from build123d import *

# Parameters (mm, degrees)
SKETCH1_W           = 243.588796282
SKETCH1_H           = 434.599999988
BOSS_EXTRUDE1_DEPTH = 12.7
CUT_EXTRUDE1_REACH  = 273.182
SKETCH2_W           = 141.287862113
SKETCH2_H           = 32.775
CUT_EXTRUDE2_REACH  = 273.182
HOLE1_D             = 3.175
HOLE1_DEPTH         = 38.1
HOLE1_CSINK_D       = 10.16
HOLE1_CSINK_ANGLE   = 82
HOLE1_TIP           = 0.953866233
CUT_EXTRUDE3_REACH  = 273.182
SKETCH6_W           = 31.75
SKETCH6_H           = 90.274999997


with BuildPart() as part:
    # Sketch1 → Boss-Extrude1 (new body)
    with BuildSketch(Plane.XY):
        with Locations((39.942597436, 0)):
            Rectangle(SKETCH1_W, SKETCH1_H)
    extrude(amount=BOSS_EXTRUDE1_DEPTH)

    # Sketch2 → Cut-Extrude1 (cut, up to next)
    with BuildSketch(Plane(origin=(0, 0, 0), x_dir=(-1, 0, 0), z_dir=(0, 0, -1)), mode=Mode.PRIVATE) as cut_extrude1_sk1:
        with Locations((11.207869649, 200.912499994)):
            Rectangle(SKETCH2_W, SKETCH2_H)
    cut_extrude1_tool1 = extrude(cut_extrude1_sk1.sketch, amount=-CUT_EXTRUDE1_REACH, mode=Mode.PRIVATE) & part.part
    # Sketch2 → Cut-Extrude1 (cut, up to next)
    with BuildSketch(Plane(origin=(0, 0, 0), x_dir=(-1, 0, 0), z_dir=(0, 0, -1)), mode=Mode.PRIVATE) as cut_extrude1_sk2:
        with Locations((11.207869649, -200.912499994)):
            Rectangle(SKETCH2_W, SKETCH2_H)
    cut_extrude1_tool2 = extrude(cut_extrude1_sk2.sketch, amount=-CUT_EXTRUDE1_REACH, mode=Mode.PRIVATE) & part.part
    add(cut_extrude1_tool1.solids().sort_by_distance((-11.20787, 200.9125, 0))[0], mode=Mode.SUBTRACT)
    add(cut_extrude1_tool2.solids().sort_by_distance((-11.20787, -200.9125, 0))[0], mode=Mode.SUBTRACT)

    # Sketch3 → Cut-Extrude2 (cut, up to next)
    with BuildSketch(Plane.XY.offset(12.7), mode=Mode.PRIVATE) as cut_extrude2_sk1:
        Polygon((62.611061408, 94.249999997), (-56.451800705, 94.249999997), (-56.451800705, 184.524999994), (-81.851800705, 184.524999994), (-81.851800705, 94.249999997), (-85.026800705, 94.249999997), (-85.026800705, -94.249999997), (-81.851800705, -94.249999997), (-81.851800705, -184.524999994), (-56.451800705, -184.524999994), (-56.451800705, -94.249999997), (62.611061408, -94.249999997), align=None)
    cut_extrude2_tool1 = extrude(cut_extrude2_sk1.sketch, amount=-CUT_EXTRUDE2_REACH, mode=Mode.PRIVATE) & part.part
    add(cut_extrude2_tool1.solids().sort_by_distance((-19.405412, 0, 12.7))[0], mode=Mode.SUBTRACT)

    # Hole1
    with Locations(Plane(origin=(449.828463103, 0, 12.7), x_dir=(0, 1, 0), z_dir=(0, 0, 1))):
        with Locations((-108.649999997, 332.89193461), (108.649999997, 332.89193461), (207.774999994, 332.89193461), (174.999999994, 448.336332751), (135.266666663, 384.042401694), (176.283333328, 384.042401694), (-174.999999994, 448.336332751), (-135.266666663, 384.042401694), (-176.283333328, 384.042401694), (-207.774999994, 332.89193461)):
            CounterSinkHole(HOLE1_D / 2, HOLE1_CSINK_D / 2, depth=HOLE1_DEPTH, counter_sink_angle=HOLE1_CSINK_ANGLE)
            with Locations((0, 0, -(HOLE1_DEPTH + HOLE1_TIP / 2))):  # 118° drill point
                Cone(0, HOLE1_D / 2, HOLE1_TIP, mode=Mode.SUBTRACT)

    # Sketch6 → Cut-Extrude3 (cut, up to next)
    with BuildSketch(Plane.XY.offset(12.7), mode=Mode.PRIVATE) as cut_extrude3_sk1:
        with Locations((-40.576800705, 139.387499996)):
            Rectangle(SKETCH6_W, SKETCH6_H)
    cut_extrude3_tool1 = extrude(cut_extrude3_sk1.sketch, amount=-CUT_EXTRUDE3_REACH, mode=Mode.PRIVATE) & part.part
    # Sketch6 → Cut-Extrude3 (cut, up to next)
    with BuildSketch(Plane.XY.offset(12.7), mode=Mode.PRIVATE) as cut_extrude3_sk2:
        with Locations((-40.576800705, -139.387499996)):
            Rectangle(SKETCH6_W, SKETCH6_H)
    cut_extrude3_tool2 = extrude(cut_extrude3_sk2.sketch, amount=-CUT_EXTRUDE3_REACH, mode=Mode.PRIVATE) & part.part
    add(cut_extrude3_tool1.solids().sort_by_distance((-40.576801, 139.3875, 12.7))[0], mode=Mode.SUBTRACT)
    add(cut_extrude3_tool2.solids().sort_by_distance((-40.576801, -139.3875, 12.7))[0], mode=Mode.SUBTRACT)


solid = part.part
Work out the finished part from the listing and answer in its coordinate system (mm). A direction names the side the tool comes from. Round coordinates to 2 decimals unless told otherwise and drop trailing zeros. Loops run counter-clockwise (first coordinate to the right, second up) from the corner with the lowest first, then second, coordinate; pieces in that order, holes last. Notation, with made-up numbers: (55, -29) - (114, -29) arc R17 cw to (114, -15) - close; hole circle Ø1 at (77, 70.25). An arc over 180 degrees is marked (long way). One line per item, written item: value.
Q1. Each of these flat-tipped pins is pushed along its axis until it touches: pin 1 Ø5 at (x, y) = (116.94, 108.65) entering from +Z; pin 2 Ø2.5 at (x, y) = (1.49, 175) entering from +Z; pin 3 Ø4 at (y, z) = (-198, 6) entering from -X; pin 4 Ø6.5 at (x, z) = (-1.5, 6.5) entering from +Y (3 decimals). Where does it stop, or does it pass through?
Check values:
pin 1: z = 9.74
pin 2: through
pin 3: x = 59.44
pin 4: y = 184.525
Q2. For faces 1 (the flat face through (20, 94.25, 6)), 2 (the flat face through (18, -184.525, 6)), 3 (the flat face through (18, 184.525, 6)), determine the directions among +Z, -Z, +X, -X, +Y, -Y from which every point of the face is accessible in a straight line to the end or side of a thin tool.
Check values:
face 1: +Z, -Z, -X
face 2: +Z, -Z, -X, -Y
face 3: +Z, -Z, -X, +Y
Q3. Straight lines are drawn through the part: probe 1 along Y at (x, z) = (55, 11) (3 decimals); probe 2 along X at (y, z) = (-40, 10); probe 3 along X at (y, z) = (191.5, 10.25). For each, find the intervals that lie inside material, in ascending order.
Check values:
probe 1: -184.525 to -94.25, 94.25 to 184.525
probe 2: 62.61 to 161.74
probe 3: 59.44 to 161.74
Q4. Find section A-A on y = 33. Give the vertices of the cut face in (x, z), and give its area (3 significant figures).
Check values:
outline: (62.61, 0) - (161.74, 0) - (161.74, 12.7) - (62.61, 12.7) - close
area: 1,260 mm2
Q5. The mould has two halves that part along X. Classify faces 4 (the flat face through (88, 3, 12.7)), 5 (the conical face through (67.345, 175.473, 8.877)), 6 (the flat face through (59.436, 201, 6)): +X half, -X half, draft (parallel to the pull), parting line (faces both ways), or undercut.
Check values:
face 4: draft
face 5: undercut
face 6: -X half
Q6. Find section B-B on z = 4. State how many separate pieces and enclosed holes the cut face has, and give its area (3 significant figures).
Check values:
separate pieces: 1
enclosed holes: 10
area: 59,000 mm2
